Source: CAD feature listing. Evaluate the final solid. Frame: model axes, mm. Face numbers are marked on the shaded views. Coordinates: 2 decimals unless noted, no trailing zeros. Answer as a JSON object with one key per item and string values. Group by question number.
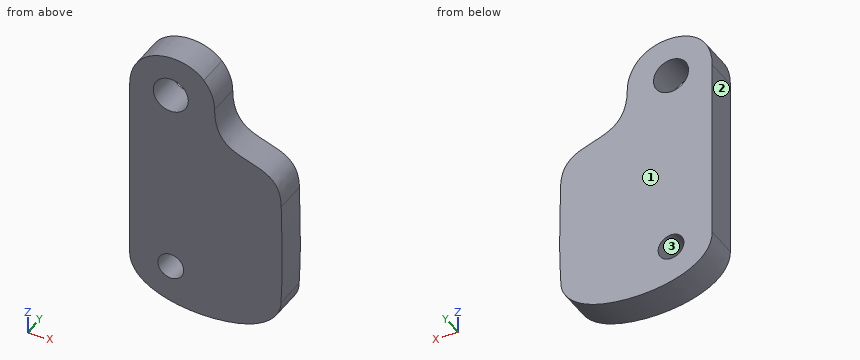
from build123d import *

# Parameters (mm, degrees)
SKETCH1_R           = 1.7
SKETCH1_R_2         = 1.25
BOSS_EXTRUDE1_DEPTH = 3.175


with BuildPart() as part:
    # Sketch1 → Boss-Extrude1 (new body)
    with BuildSketch(Plane(origin=(0, 0, 0), x_dir=(1, 0, 0), z_dir=(0, 1, 0))):
        with BuildLine():
            Line((-7.40608976, 8.047333881), (-7.40608976, -9.667484989))
            add(Edge.make_bspline(
                [(-7.40608976, -9.667484989), (-7.427440527, -14.359265116), (-2.104976514, -14.822390535), (-0.211157807, -12.684787438)],
                knots=[3, 3, 3, 3, 4, 4, 4, 4], degree=3))
            add(Edge.make_bspline(
                [(-0.211157807, -12.684787438), (0.454759152, -11.961542687), (0.830932646, -10.979054864), (0.834200784, -9.953266472)],
                knots=[4, 4, 4, 4, 5, 5, 5, 5], degree=3))
            add(Edge.make_bspline(
                [(0.834200784, -9.953266472), (0.847614911, -3.759244356), (7.276744818, -7.46221529), (7.299751606, -2.008967061)],
                knots=[5, 5, 5, 5, 6, 6, 6, 6], degree=3))
            add(Edge.make_bspline(
                [(7.299751606, -2.008967061), (7.310026672, 0.456281555), (7.523736335, 3.752134489), (7.276744819, 8.147321264)],
                knots=[6, 6, 6, 6, 7, 7, 7, 7], degree=3))
            add(Edge.make_bspline(
                [(7.276744819, 8.147321264), (7.287246129, 9.173061108), (6.632340018, 10.163694097), (5.456847891, 10.900933881)],
                knots=[7, 7, 7, 7, 8, 8, 8, 8], degree=3))
            add(Edge.make_bspline(
                [(5.456847891, 10.900933881), (2.10699507, 13.081407092), (-7.386860521, 12.739250307), (-7.40608976, 8.047333881)],
                knots=[8, 8, 8, 8, 9, 9, 9, 9], degree=3))
        make_face()
        with Locations(Location((-3.413173976, -9.953168809, 0), (0, 0, 270))):
            Circle(SKETCH1_R, mode=Mode.SUBTRACT)
        with Locations(Location((-3.413271461, 8.147321264, 0), (0, 0, 270))):
            Circle(SKETCH1_R_2, mode=Mode.SUBTRACT)
    extrude(amount=BOSS_EXTRUDE1_DEPTH)


solid = part.part
1. Section query A-A on x = -2.5. State how many separate pieces and enclosed holes the cut face has, then the cut area to 3 significant figures.
2. Ray query, L1, parallel to X at y = 0.25, z = -4.5; L2, parallel to Z at x = -4, y = 1.3; L3, parallel to X at y = 0.8, z = 9. Return the intervals inside material, ascending.
3. Mould query, pull axis X, two halves, no side actions, for the marked faces 1, 2 and 3. Classes: pulls with the +X half, pulls with the -X half, needs draft (parallel to the pull), parting line crosses it, or undercut.
4. Pin query (flat end, axial travel): pin 1 Ø4 at (x, z) = (-3.41, 9.95) entering from +Y (3 decimals); pin 2 Ø2 at (x, z) = (-3.41, -8.15) entering from -Y. Return the tip coordinate at first contact, or that it passes through.
Solved:
{
 "1": {"separate pieces": "3", "enclosed holes": "0", "area": "67.6 mm^2"},
 "2": {"L1": "-7.41 to 7.39", "L2": "-11.66 to -9.25, -7.04 to 8.36, 11.55 to 13.85", "L3": "-7.41 to -4.82, -2.01 to 0.89"},
 "3": {"face 1": "needs draft", "face 2": "pulls with the -X half", "face 3": "undercut"},
 "4": {"pin 1": "y = 3.175", "pin 2": "through"}
}
